Check sheet for the drawn part. Datum: minimum x, y, z corner. Units: mm. A direction names the side the tool comes from. Round coordinates to 2 decimals unless told otherwise and drop trailing zeros. Write each loop counter-clockwise with the first axis right and the second up, starting at its lowest first coordinate (ties: lowest second). Pieces come first, ordered by that corner, then holes. Notation, with made-up numbers: M 66,-8 L 74,-8 A19 ccw 74,-3 Z; hole C 66.5,12 d5. An arc over 180 degrees is marked long. One line per item, written item: value.
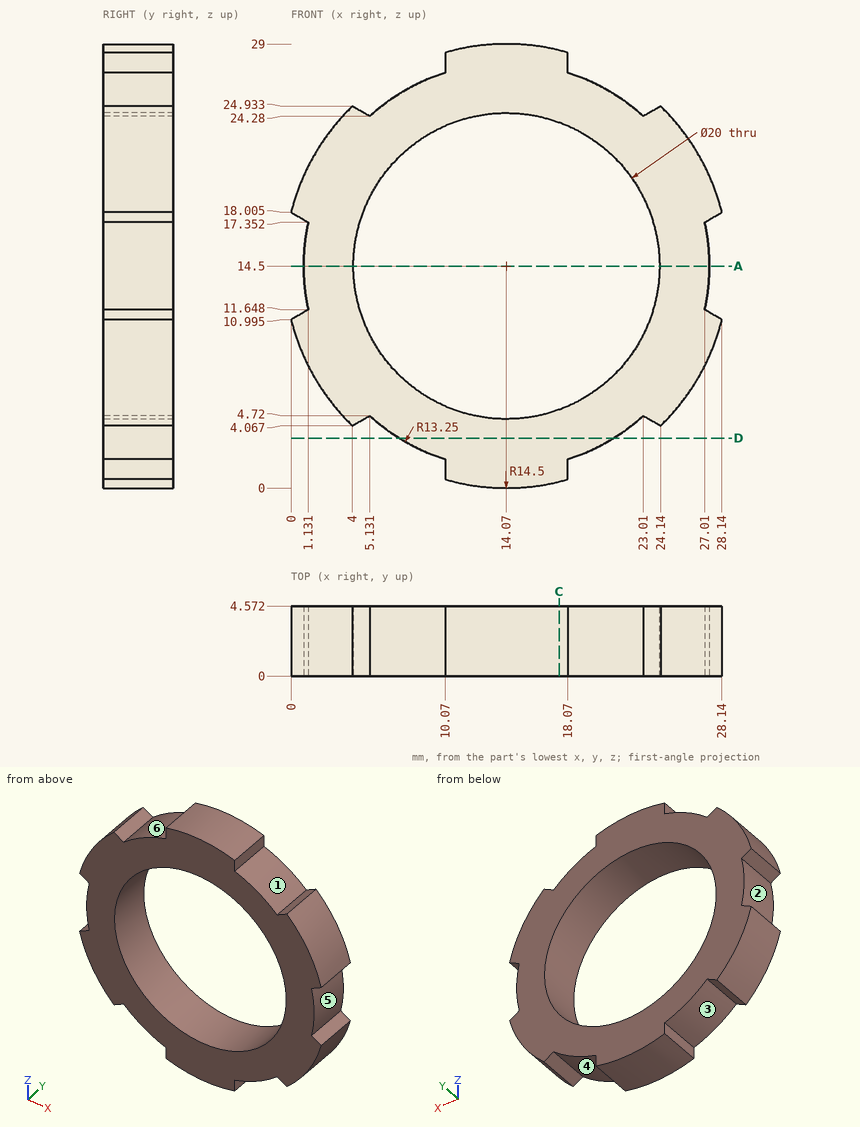
Q1. Sectioned sample at C-C on x = 17.5. Enter the section's corners in (y, z).
Completed:
outline: M 0,0.41 L 4.57,0.41 L 4.57,5.11 L 0,5.11 Z; M 0,23.89 L 4.57,23.89 L 4.57,28.59 L 0,28.59 Z
Q2. Sectioned sample at D-D on z = 3.25. Enter the section's corners in (x, y), and give its area (3 significant figures).
Completed:
outline: M 7.07,0 L 21.07,0 L 21.07,4.57 L 7.07,4.57 Z
area: 64.0 mm^2
Q3. Depth check by flat-ended pin: P1, Ø1, axis at y = 2.5, z = 28, coming from the -X side; P2, Ø1, axis at y = 1.5, z = 28, coming from the +X side; P3, Ø1.5, axis at x = 12, y = 3.5, coming from the +Z side. Enter the tip coordinate at first touch or a pass-through.
Completed:
P1: x = 10.07
P2: x = 18.07
P3: z = 28.94
Q4. Draft check along Z on the marked faces 1, 2 and 3. Enter one of: pulls with the +Z half, pulls with the -Z half, needs draft (parallel to the pull), parting line crosses it, or undercut.
Completed:
face 1: pulls with the +Z half
face 2: undercut
face 3: pulls with the -Z half
Q5. Scan lines: line 1 (X direction, y = 1.6, z = 14.5); line 2 (Z direction, x = 22.75, y = 3.3) (1 decimal); line 3 (Z direction, x = 13, y = 4.25). Record each from-to range of solid material in increasing order. Write a range as [from, to].
Completed:
line 1: [0.82, 4.07], [24.07, 27.32]
line 2: [4.5, 9.5], [19.5, 24.5]
line 3: [0.04, 4.56], [24.44, 28.96]
Q6. Access from +Z, -Z, +X, -X, +Y, -Y to the whole of each face (thin tool, end or side, straight path). Record for the marked faces 4, 5 and 6.
Completed:
face 4: -Z, +Y, -Y
face 5: +X, +Y, -Y
face 6: +Z, +Y, -Y
Q7. Sectioned sample at A-A on z = 14.5. Enter the section's corners in (x, y), and give its area (3 significant figures).
Completed:
outline: M 0.82,0 L 4.07,0 L 4.07,4.57 L 0.82,4.57 Z; M 24.07,0 L 27.32,0 L 27.32,4.57 L 24.07,4.57 Z
area: 29.7 mm^2
